from build123d import *

# Parameters (mm, degrees)
SKETCH2_W          = 1.5875
SKETCH2_H          = 6.148361062
CUT_EXTRUDE1_DEPTH = 7.9375
SKETCH3_R          = 1.55
CUT_EXTRUDE2_DEPTH = 23.082804042
SKETCH4_R          = 1.55
CUT_EXTRUDE3_DEPTH = 23.082804093
CHAMFER1_SIZE      = 0.127
SCALE1_SCALE       = 1.5


with BuildPart() as part:
    # Sketch1 → Revolve1 (revolve)
    with BuildSketch(Plane.XY, mode=Mode.PRIVATE) as revolve1_sk:
        Polygon((6.35, 0), (6.35, 7.9375), (13.49375, 7.9375), (13.49375, 11.1125), (2.38125, 11.1125), (2.38125, 0), align=None)
    revolve(revolve1_sk.sketch.rotate(Axis((0, 0, 0), (0, 1, 0)), 90), axis=Axis((0, 0, 0), (0, 1, 0)))

    # Sketch2 → Cut-Extrude1 (cut)
    with BuildSketch(Plane.XZ):
        with Locations((-6.35, 0)):
            Rectangle(SKETCH2_W, SKETCH2_H)
        with Locations((6.35, 0)):
            Rectangle(SKETCH2_W, SKETCH2_H)
    extrude(amount=-CUT_EXTRUDE1_DEPTH, mode=Mode.SUBTRACT)

    # Sketch3 → Cut-Extrude2 (cut, through all)
    with BuildSketch(Plane(origin=(0, 0, 0), x_dir=(0, 0, -1), z_dir=(1, 0, 0))):
        with Locations((0, 4.7625)):
            Circle(SKETCH3_R)
    extrude(amount=-CUT_EXTRUDE2_DEPTH, mode=Mode.SUBTRACT)

    # Sketch4 → Cut-Extrude3 (cut, through all)
    with BuildSketch(Plane(origin=(0, 11.1125, 0), x_dir=(1, 0, 0), z_dir=(0, 1, 0))):
        with Locations(Location((-7.296458098, 7.296458098, 0), (0, 0, 270))):
            Circle(SKETCH4_R)
        with Locations(Location((7.296458098, 7.296458098, 0), (0, 0, 270))):
            Circle(SKETCH4_R)
        with Locations(Location((7.296458098, -7.296458098, 0), (0, 0, 270))):
            Circle(SKETCH4_R)
        with Locations(Location((-7.296458098, -7.296458098, 0), (0, 0, 270))):
            Circle(SKETCH4_R)
    extrude(amount=-CUT_EXTRUDE3_DEPTH, mode=Mode.SUBTRACT)

    # Chamfer1
    chamfer1_edges = [part.edges().sort_by_distance(p)[0] for p in [
        (0, 0, -6.35),
        (-5.55625, 0, 0),
        (0, 0, 6.35),
        (5.55625, 0, 0),
        (0, 7.9375, 13.49375),
        (0, 11.1125, 13.49375),
    ]]
    chamfer(chamfer1_edges, length=CHAMFER1_SIZE)


with BuildPart() as part_1:
    # Scale1: scaled about (0.039762261, 7.732974778, -1.52e-07)
    add(part.part.scale(SCALE1_SCALE).moved(Location((-0.019881131, -3.866487389, 7.6e-08))))


solid = part_1.part
Check sheet for the modelled part. Datum: model origin and axes. Units: mm. A direction names the side the tool comes from. Give positions to 0.01 mm unless a question says otherwise; leave off trailing zeros. Order: outer loops, then holes, each group sorted by start corner. A loop starts at its lowest first (then second) coordinate and runs counter-clockwise, first axis right, second up. Notation, with made-up numbers: (71.25, 37) - (89.25, 37) arc R31 ccw to (89.25, 70) - close; hole circle Ø9 at (39, 25.5). An arc over 180 degrees is marked (long way). Answer as CSV lines item,"result".
1. Section check D-D (z = 12). State how many separate pieces and enclosed holes the cut face has, then the cut area to 3 significant figures.
Result sheet:
separate pieces,"3"
enclosed holes,"0"
area,"116 mm²"
2. Go/stop test with flat-tipped pins: P1, Ø4, axis at y = 3.28, z = 0, coming from the -X side; P2, Ø3.5, axis at x = -10.96, z = -10.94, coming from the +Y side; P3, Ø3, axis at x = 5.5, y = 7, coming from the -Z side; P4, Ø3, axis at x = 8, y = 3.5, coming from the -Z side. Record where each tip stops, or that it passes through.
Result sheet:
P1,"x = 2.94"
P2,"through"
P3,"z = -19.7"
P4,"z = -6.94"
3. Section check A-A (z = 0). Record the boundary of the cut face in (x, y), then the cut area to 3 significant figures.
Result sheet:
outline,"(-20.26, 8.23) - (-20.07, 8.04) - (-8.35, 8.04) - (-8.35, 5.6) - (-3.59, 5.6) - (-3.59, 12.8) - (-20.07, 12.8) - (-20.26, 12.61) - close; (-8.35, -3.68) - (-8.16, -3.87) - (-3.59, -3.87) - (-3.59, 0.95) - (-8.35, 0.95) - close; (3.55, -3.87) - (8.12, -3.87) - (8.31, -3.68) - (8.31, 8.04) - (20.03, 8.04) - (20.22, 8.23) - (20.22, 12.61) - (20.03, 12.8) - (3.55, 12.8) - close"
area,"250 mm²"
4. Tool access check on faces 5 (the face through (-0.162, 2.264, 9.524)), 6 (the face through (8.314, 2, 0)), 7 (the face through (0.122, 2.264, -9.524)), 8 (the face through (-5.503, 3.976, -2.218)). Record the directions out of +Z, -Z, +X, -X, +Y, -Y that give a thin tool (end or side, any length) a straight path to the whole face; none if there is none.
Result sheet:
face 5,"+Z, -Y"
face 6,"+Z, -Z, +X, -Y"
face 7,"-Z, -Y"
face 8,"-X"
5. Mould release check, pull along X, two halves, no side actions. Record for faces 1 (the face through (-6.1, 10.452, -19.306)), 2 (the face through (9, 8.04, 0)), 3 (the face through (-9.393, 10.454, -12.658)), 4 (the face through (-8.354, 0.8, -0.1)): released by +X, released by -X, zero draft, split by the parting line, or undercut.
Result sheet:
face 1,"split by the parting line"
face 2,"zero draft"
face 3,"undercut"
face 4,"released by -X"
6. Scan lines: probe 1 along Y at (x, z) = (-6.5, 0); probe 2 along X at (y, z) = (10.75, 9.5); probe 3 along Y at (x, z) = (-14, -11). Record each from-to range of solid material in increasing order. Write a range as from..to.
Result sheet:
probe 1,"-3.87..0.95, 5.6..12.8"
probe 2,"-17.89..-12.79, -9.14..9.1, 12.75..17.85"
probe 3,"8.04..12.8"
